```python
from build123d import *

# Parameters (mm, degrees)
IZIM1_R                     = 8
Y_KSEKLIK_EKSTR_ZYON1_DEPTH = 12
Y_KSEKLIK_EKSTR_ZYON2_DEPTH = 46
IZIM4_R                     = 15
KES_EKSTR_ZYON1_DEPTH       = 10
IZIM5_R                     = 10
KES_EKSTR_ZYON2_DEPTH       = 114.846387734
FEDER7_REACH                = 101.057
IZIM16_WALL_W               = 253.965251844
IZIM16_WALL_H               = 8


with BuildPart() as part:
    # Çizim1 → Yükseklik-Ekstrüzyon1 (new body)
    with BuildSketch(Plane(origin=(0, 0, 0), x_dir=(1, 0, 0), z_dir=(0, 1, 0))):
        with BuildLine():
            Line((48, 0), (-48, 0))
            ThreePointArc((-48, 0), (-59.313708499, 4.686291501), (-64, 16))
            Line((-64, 16), (-64, 49))
            Line((-64, 49), (-64, 65))
            ThreePointArc((-64, 65), (-59.313708499, 76.313708499), (-48, 81))
            Line((-48, 81), (48, 81))
            ThreePointArc((48, 81), (59.313708499, 76.313708499), (64, 65))
            Line((64, 65), (64, 49))
            Line((64, 49), (64, 16))
            ThreePointArc((64, 16), (59.313708499, 4.686291501), (48, 0))
        make_face()
        with Locations(Location((-48, 65, 0), (0, 0, 270))):
            Circle(IZIM1_R, mode=Mode.SUBTRACT)
        with Locations(Location((-48, 16, 0), (0, 0, 270))):
            Circle(IZIM1_R, mode=Mode.SUBTRACT)
        with Locations(Location((48, 65, 0), (0, 0, 270))):
            Circle(IZIM1_R, mode=Mode.SUBTRACT)
        with Locations(Location((48, 16, 0), (0, 0, 270))):
            Circle(IZIM1_R, mode=Mode.SUBTRACT)
    extrude(amount=Y_KSEKLIK_EKSTR_ZYON1_DEPTH)

    # Çizim2 → Yükseklik-Ekstrüzyon2 (add)
    with BuildSketch(Plane(origin=(0, 12, 0), x_dir=(1, 0, 0), z_dir=(0, 1, 0))):
        with BuildLine():
            Line((-20, 62.860679775), (-20, 40.5))
            Line((-20, 40.5), (-20, 18.139320225))
            ThreePointArc((-20, 18.139320225), (30, 40.5), (-20, 62.860679775))
        make_face()
    extrude(amount=Y_KSEKLIK_EKSTR_ZYON2_DEPTH)

    # Çizim4 → Kes-Ekstrüzyon1 (cut)
    with BuildSketch(Plane(origin=(0, 58, 0), x_dir=(1, 0, 0), z_dir=(0, 1, 0))):
        with Locations(Location((0, 40.5, 0), (0, 0, 270))):
            Circle(IZIM4_R)
    extrude(amount=-KES_EKSTR_ZYON1_DEPTH, mode=Mode.SUBTRACT)

    # Çizim5 → Kes-Ekstrüzyon2 (cut, through all)
    with BuildSketch(Plane(origin=(0, 48, 0), x_dir=(1, 0, 0), z_dir=(0, 1, 0))):
        with Locations(Location((0, 40.5, 0), (0, 0, 270))):
            Circle(IZIM5_R)
    extrude(amount=-KES_EKSTR_ZYON2_DEPTH, mode=Mode.SUBTRACT)

    # Çizim16 wall → Feder7 (add, up to next)
    with BuildSketch(Plane(origin=(-34, 35, -32.5), x_dir=(0.519946946896, 0.854198555614, 0), z_dir=(-0.854198555614, 0.519946946896, 0)), mode=Mode.PRIVATE) as feder7_sk1:
        Rectangle(IZIM16_WALL_W, IZIM16_WALL_H)
    feder7_tool1 = extrude(feder7_sk1.sketch, amount=-FEDER7_REACH, mode=Mode.PRIVATE) - part.part
    add(feder7_tool1.solids().sort_by_distance((-34, 35, -32.5))[0])


solid = part.part
```
CAD build for the part. Positions are in the model's coordinates, mm. A direction names the side the tool comes from. Round coordinates to 2 decimals unless told otherwise and drop trailing zeros. Loops run counter-clockwise (first coordinate to the right, second up) from the corner with the lowest first, then second, coordinate; pieces in that order, holes last. Notation, with made-up numbers: (82.5, 64) - (92.5, 64) arc R9 ccw to (92.5, 70) - close; hole circle Ø4 at (-26.75, 31). An arc over 180 degrees is marked (long way). Return JSON: item names as keys, results as strings. Group by question number.
Q1. Band-saw the part on D-D on y = 5.5. Give the cut face in (x, z), plus the area to 3 significant figures.
Q2. Two-plate mould, pull along Z, no slides. Class faces 1 (the face through (55.932, 5.916, -17.041)), 2 (the face through (16, 58, -41)), 3 (the face through (1, 6, 0)): +Z half, -Z half, draft (parallel to the pull), parting line (faces both ways), or undercut.
Q3. Band-saw the part on A-A on z = -40.5. Give the cut face in (x, y), plus the area to 3 significant figures.
Q4. Band-saw the part on C-C on y = 18.5. Give the cut face in (x, z), plus the area to 3 significant figures.
Q5. Flat gauge pins, fed straight in: pin 1 Ø8 at (x, y) = (10.5, 32.5) entering from -Z; pin 2 Ø8 at (y, z) = (28, -55) entering from -X; pin 3 Ø6 at (y, z) = (41.5, -37) entering from -X. Where does each tip first touch, or does it go through?
Q6. Band-saw the part on B-B on x = 0. Give the cut face in (y, z).
Q7. Drill centre lines: line 1 along X through (y, z) = (8, -16); line 2 along Y through (x, z) = (-43, -25); line 3 along Z through (x, y) = (-45, 5). Where is each one in solid material? Low to high. Write a range as [from, to].
Q8. Tool access for faces 4 (the face through (-30, 25, -28.5)), 5 (the face through (0.44, 24.34, -50.49)), 6 (the face through (-28, 12, -41)): list every direction of +Z, -Z, +X, -X, +Y, -Y with a clear straight run to the whole face (end or side of a thin tool).
Solutions:
{
 "1": {"outline": "(-64, -65) arc R16 ccw to (-48, -81) - (48, -81) arc R16 ccw to (64, -65) - (64, -16) arc R16 ccw to (48, 0) - (-48, 0) arc R16 ccw to (-64, -16) - close; hole circle Ø16 at (-48, -65); hole circle Ø16 at (-48, -16); hole circle Ø20 at (0, -40.5); hole circle Ø16 at (48, -65); hole circle Ø16 at (48, -16)", "area": "9,030 mm^2"},
 "2": {"face 1": "undercut", "face 2": "draft", "face 3": "+Z half"},
 "3": {"outline": "(-64, 0) - (-10, 0) - (-10, 48) - (-15, 48) - (-15, 58) - (-20, 58) - (-20, 12) - (-64, 12) - close; (10, 0) - (64, 0) - (64, 12) - (30, 12) - (30, 58) - (15, 58) - (15, 48) - (10, 48) - close", "area": "2,580 mm^2"},
 "4": {"outline": "(-44.04, -36.5) - (-20, -36.5) - (-20, -62.86) arc R30 ccw (long way) to (-20, -18.14) - (-20, -28.5) - (-44.04, -28.5) - close; hole circle Ø20 at (0, -40.5)", "area": "2,400 mm^2"},
 "5": {"pin 1": "stops at z = -69.79", "pin 2": "stops at x = -20", "pin 3": "stops at x = -31.84"},
 "6": {"outline": "(0, -81) - (12, -81) - (12, -70.5) - (58, -70.5) - (58, -55.5) - (48, -55.5) - (48, -50.5) - (0, -50.5) - close; (0, -30.5) - (48, -30.5) - (48, -25.5) - (58, -25.5) - (58, -10.5) - (12, -10.5) - (12, 0) - (0, 0) - close"},
 "7": {"line 1": "x = [-64, -56], [-40, 40], [56, 64]", "line 2": "y = [0, 12]", "line 3": "z = [-81, -72.42], [-57.58, -23.42], [-8.58, 0]"},
 "8": {"face 4": "+Z, -X, +Y", "face 5": "+Y, -Y", "face 6": "+Y"}
}
